Can you work these out from the model? Positions are in its coordinate system, mm. A direction names the side the tool comes from. Coordinates: 2 decimals unless noted, no trailing zeros. Order: outer loops, then holes, each group sorted by start corner. A loop starts at its lowest first (then second) coordinate and runs counter-clockwise, first axis right, second up. Notation, with made-up numbers: (21, 17) -> (60, 17) arc R11 ccw to (60, 36) -> close; hole circle Ø9 at (56.5, 24.25). An arc over 180 degrees is marked (long way). Answer in a Markdown table with one row per item. Add a question column.
1. Imagine slicing it at D-D on y = 84. Write out the boundary of the cut face in (x, z), plus the area to 3 significant figures.
2. Imagine slicing it at B-B on y = 176. Write out the boundary of the cut face in (x, z).
3. Will these pins go through, and if not, where does the flat tip stop? pin 1 (4 mm diameter, centred on x = 28, z = -14, fed in from +Y); pin 2 (4 mm diameter, centred on x = -19, z = 56.5, fed in from +Y); pin 3 (15 mm diameter, centred on x = 5.5, y = 45, fed in from -Z).
4. If I drill on line 1 along Z through (x, y) = (-12, 175.5); line 2 along X through (y, z) = (187.96, -73.55); line 3 along Y through (x, z) = (-43.5, 7), over which ranges is the centre line in solid material (lowest first)? Write a range as [from, to].
5. Imagine slicing it at C-C on z = 0. Write out the boundary of the cut face in (x, y), plus the area to 3 significant figures.
6. On a 3-axis mill with a long thin cutter (end or side, diameter ignored), from which of +Z, -Z, +X, -X, +Y, -Y can I reach the whole of each face in a straight line? I mean faces 5 (the face through (-39, 152.4, -1)), 6 (the face through (0, 38, 76.2)), 7 (the face through (13.65, 59.52, -51.96)), 8 (the face through (0.4, 143.51, -0.64)), 9 (the face through (-16.604, 200.855, 73.696)). Say none if no direction works.
7. We'd pull the mould along X, two halves only. Please class faces 1 (the face through (1, 189, 71.12)), 2 (the face through (-50.8, 150, -1)), 3 (the face through (23.463, 28.372, 52.634)), 4 (the face through (0, 38, -76.2)): pulls with the +X half, pulls with the -X half, needs draft (parallel to the pull), parting line crosses it, or undercut.
8. Imagine slicing it at A-A on z = 66.5. Write out the boundary of the cut face in (x, y), plus the area to 3 significant figures.
from build123d import *

# Parameters (mm, degrees)
SKETCH1_R           = 38.1
BOSS_EXTRUDE1_DEPTH = 127
SKETCH3_R           = 25.4
BOSS_EXTRUDE2_DEPTH = 152.4
SKETCH4_W           = 101.6
SKETCH4_H           = 152.4
BOSS_EXTRUDE3_DEPTH = 10.16
SKETCH5_W           = 101.6
SKETCH5_H           = 30.48
BOSS_EXTRUDE4_DEPTH = 101.6
CUT_EXTRUDE1_DEPTH  = 101.6
SKETCH8_R           = 44.45
SKETCH8_R_2         = 9.525
CUT_EXTRUDE3_DEPTH  = 5.08
BOSS_EXTRUDE6_START = 2.54
SKETCH8_6_R         = 9.525
BOSS_EXTRUDE6_DEPTH = 2.54
BOSS_EXTRUDE7_DEPTH = 121.92
SKETCH11_R          = 38.1
CUT_EXTRUDE5_DEPTH  = 12.7


with BuildPart() as part:
    # Sketch1 → Boss-Extrude1 (new body)
    with BuildSketch(Plane(origin=(0, 0, 0), x_dir=(1, 0, 0), z_dir=(0, 1, 0))):
        with Locations(Location((0, 0, 0), (0, 0, 270))):
            Circle(SKETCH1_R)
    extrude(amount=BOSS_EXTRUDE1_DEPTH)

    # Sketch3 → Boss-Extrude2 (add)
    with BuildSketch(Plane.XY.offset(76.2)):
        with Locations((0, 38.1)):
            Circle(SKETCH3_R)
    extrude(amount=-BOSS_EXTRUDE2_DEPTH)

    # Sketch4 → Boss-Extrude3 (add)
    with BuildSketch(Plane(origin=(0, 127, 0), x_dir=(1, 0, 0), z_dir=(0, 1, 0))):
        Rectangle(SKETCH4_W, SKETCH4_H)
    extrude(amount=BOSS_EXTRUDE3_DEPTH)

    # Sketch5 → Boss-Extrude4 (add)
    with BuildSketch(Plane(origin=(0, 137.16, 0), x_dir=(1, 0, 0), z_dir=(0, 1, 0))):
        with Locations((0, 60.96)):
            Rectangle(SKETCH5_W, SKETCH5_H)
    boss_extrude4 = extrude(amount=BOSS_EXTRUDE4_DEPTH)

    # Sketch7 → Cut-Extrude1 (cut)
    with BuildSketch(Plane(origin=(0, 0, -76.2), x_dir=(-1, 0, 0), z_dir=(0, 0, -1))):
        with BuildLine():
            ThreePointArc((-50.8, 187.96), (-35.92102454, 223.881024429), (-1.57e-07, 238.76))
            Line((-1.57e-07, 238.76), (-50.8, 238.76))
            Line((-50.8, 238.76), (-50.8, 187.96))
        make_face()
        with BuildLine():
            Line((50.8, 187.96), (50.8, 238.76))
            Line((50.8, 238.76), (-1.57e-07, 238.76))
            ThreePointArc((-1.57e-07, 238.76), (35.921024429, 223.88102454), (50.8, 187.96))
        make_face()
    cut_extrude1 = extrude(amount=-CUT_EXTRUDE1_DEPTH, mode=Mode.SUBTRACT)

    # Sketch8 → Cut-Extrude3 (cut)
    with BuildSketch(Plane(origin=(0, 0, -76.2), x_dir=(-1, 0, 0), z_dir=(0, 0, -1))):
        with Locations((0, 187.96)):
            Circle(SKETCH8_R)
        with Locations((-28.554667319, 193.031059488)):
            Circle(SKETCH8_R_2, mode=Mode.SUBTRACT)
        with Locations((9.885667319, 160.695402961)):
            Circle(SKETCH8_R_2, mode=Mode.SUBTRACT)
        with Locations((18.669, 210.153537551)):
            Circle(SKETCH8_R_2, mode=Mode.SUBTRACT)
    cut_extrude3 = extrude(amount=-CUT_EXTRUDE3_DEPTH, mode=Mode.SUBTRACT)

    # Sketch8<6> → Boss-Extrude6 (add)
    with BuildSketch(Plane(origin=(0, 0, -76.2), x_dir=(-1, 0, 0), z_dir=(0, 0, -1)).offset(BOSS_EXTRUDE6_START)):
        with Locations((-28.554667319, 193.031059488)):
            Circle(SKETCH8_6_R)
        with Locations((9.885667319, 160.695402961)):
            Circle(SKETCH8_6_R)
    boss_extrude6 = extrude(amount=-BOSS_EXTRUDE6_DEPTH)

    # Mirror2: Boss-Extrude4, Cut-Extrude1, Cut-Extrude3, Boss-Extrude6 across plane
    add(boss_extrude4.mirror(Plane.XY))
    add(cut_extrude1.mirror(Plane.XY), mode=Mode.SUBTRACT)
    add(cut_extrude3.mirror(Plane.XY), mode=Mode.SUBTRACT)
    add(boss_extrude6.mirror(Plane.XY))

    # Sketch10 → Boss-Extrude7 (add)
    with BuildSketch(Plane(origin=(0, 0, -76.2), x_dir=(-1, 0, 0), z_dir=(0, 0, -1))):
        with BuildLine():
            Line((-50.8, 152.4), (-26.67, 152.4))
            ThreePointArc((-26.67, 152.4), (0, 143.51), (26.67, 152.4))
            Line((26.67, 152.4), (50.8, 152.4))
            Line((50.8, 152.4), (50.8, 127))
            Line((50.8, 127), (-50.8, 127))
            Line((-50.8, 127), (-50.8, 152.4))
        make_face()
    extrude(amount=-BOSS_EXTRUDE7_DEPTH)

    # Sketch11 → Cut-Extrude5 (cut)
    with BuildSketch(Plane.XZ):
        with Locations(Location((0, 0, 0), (0, 0, 90))):
            Circle(SKETCH11_R)
    extrude(amount=-CUT_EXTRUDE5_DEPTH, mode=Mode.SUBTRACT)


solid = part.part
Answers follow:
| question | item | result |
|---|---|---|
| 1 | outline | circle Ø76.2 at (0, 0) |
| 1 | area | 4,560 mm² |
| 2 | outline | (-50.8, -76.2) -> (-42.81, -76.2) -> (-42.81, -71.12) -> (42.81, -71.12) -> (42.81, -76.2) -> (50.8, -76.2) -> (50.8, -45.72) -> (-50.8, -45.72) -> close; (-50.8, 45.72) -> (50.8, 45.72) -> (50.8, 76.2) -> (42.81, 76.2) -> (42.81, 71.12) -> (-42.81, 71.12) -> (-42.81, 76.2) -> (-50.8, 76.2) -> close |
| 3 | pin 1 | stops at y = 152.4 |
| 3 | pin 2 | stops at y = 235.83 |
| 3 | pin 3 | stops at z = -76.2 |
| 4 | line 1 | z = [-71.12, -45.72], [45.72, 71.12] |
| 4 | line 2 | x = [-50.8, -44.45], [20.49, 36.62], [44.45, 50.8] |
| 4 | line 3 | y = [127, 152.4] |
| 5 | outline | (-50.8, 127) -> (-38.1, 127) -> (-38.1, 12.7) -> (38.1, 12.7) -> (38.1, 127) -> (50.8, 127) -> (50.8, 152.4) -> (26.67, 152.4) arc R44.45 cw to (-26.67, 152.4) -> (-50.8, 152.4) -> close |
| 5 | area | 11,000 mm² |
| 6 | face 5 | +X, -X, +Y |
| 6 | face 6 | +Z, +X, -X, -Y |
| 6 | face 7 | -Z |
| 6 | face 8 | +Y |
| 6 | face 9 | +Z |
| 7 | face 1 | undercut |
| 7 | face 2 | pulls with the -X half |
| 7 | face 3 | parting line crosses it |
| 7 | face 4 | needs draft |
| 8 | outline | (-50.8, 127) -> (50.8, 127) -> (50.8, 187.96) arc R50.8 ccw to (-50.8, 187.96) -> close; circle Ø50.8 at (0, 38.1) |
| 8 | area | 12,300 mm² |
